```python
from build123d import *

# Parameters (mm, degrees)
SKETCH_1_R          = 18.5
SKETCH_1_R_2        = 6
EXTRUDE_1_DEPTH     = 14
SKETCH_2_R          = 18.5
SKETCH_2_R_2        = 17.3
CUT_EXTRUDE_1_DEPTH = 2.2
SKETCH_2_2_R        = 18.5
SKETCH_2_2_R_2      = 17.3
CUT_EXTRUDE_2_DEPTH = 0.8
SKETCH_2_4_R        = 18.5
SKETCH_2_4_R_2      = 17.3
CUT_EXTRUDE_3_DEPTH = 4
SKETCH_2_6_R        = 18.5
SKETCH_2_6_R_2      = 17.3
CUT_EXTRUDE_5_DEPTH = 3


with BuildPart() as part:
    # Sketch 1 → Extrude 1 (new body)
    with BuildSketch(Plane.XY):
        Circle(SKETCH_1_R)
        Circle(SKETCH_1_R_2, mode=Mode.SUBTRACT)
    extrude(amount=EXTRUDE_1_DEPTH)

    # Sketch 2 → Cut-Extrude 1 (cut)
    with BuildSketch(Plane.XY.offset(7.7)):
        Circle(SKETCH_2_R)
        Circle(SKETCH_2_R_2, mode=Mode.SUBTRACT)
    extrude(amount=-CUT_EXTRUDE_1_DEPTH, mode=Mode.SUBTRACT)

    # Sketch 2_2 → Cut-Extrude 2 (cut)
    with BuildSketch(Plane.XY.offset(7.7)):
        Circle(SKETCH_2_2_R)
        Circle(SKETCH_2_2_R_2, mode=Mode.SUBTRACT)
    extrude(amount=CUT_EXTRUDE_2_DEPTH, mode=Mode.SUBTRACT)

    # Sketch 2_4 → Cut-Extrude 3 (cut)
    with BuildSketch(Plane.XY.offset(7.7)):
        Circle(SKETCH_2_4_R)
        Circle(SKETCH_2_4_R_2, mode=Mode.SUBTRACT)
    extrude(amount=-CUT_EXTRUDE_3_DEPTH, mode=Mode.SUBTRACT)

    # Sketch 2_6 → Cut-Extrude 5 (cut)
    with BuildSketch(Plane.XY.offset(7.7)):
        Circle(SKETCH_2_6_R)
        Circle(SKETCH_2_6_R_2, mode=Mode.SUBTRACT)
    extrude(amount=CUT_EXTRUDE_5_DEPTH, mode=Mode.SUBTRACT)


solid = part.part
```
Part model, mm, in its own coordinate system. A direction names the side the tool comes from. Round coordinates to 2 decimals unless told otherwise and drop trailing zeros. Loops run counter-clockwise (first coordinate to the right, second up) from the corner with the lowest first, then second, coordinate; pieces in that order, holes last. Notation, with made-up numbers: (7, 65) -> (58, 65) arc R25 cw to (58, 85) -> close; hole circle Ø8 at (-32.5, 38.5). An arc over 180 degrees is marked (long way). Use CSV: the item, a comma, the result in double quotes. Start each with the question number.
1) Wall check: L1, parallel to Z at x = 8, y = 15.5; L2, parallel to Y at x = 0, z = 6.75; L3, parallel to Y at x = 0, z = 11. Give the ranges that are in metal, low to high. Write a range as [from, to].
2) Cut at D-D, the plane x = 9.5. Write the cut outline in (y, z).
3) Cut at C-C, the plane z = 9. Write the cut outline in (x, y), plus the area to 3 significant figures.
4) Which spindle directions (+Z, -Z, +X, -X, +Y, -Y) get a long thin tool onto all of the face, cutting with end or side? Do faces 1 (the flat face through (11, -14, 3.7)), 2 (the flat face through (-4.4, 4.4, 0)). Say none if no direction does.
5) Cut at A-A, the plane y = 0. Write the cut outline in (x, z), plus the area to 3 significant figures.
6) Drop flat-ended pins along their axis: P1, Ø3, axis at x = -13.5, z = 8, coming from the -Y side; P2, Ø1, axis at y = -14.5, z = 5.5, coming from the +X side; P3, Ø6, axis at y = -8.5, z = 4, coming from the -X side. Give the stop position or say it passes through.
7) Pull direction X, two halves, no side cores. Call faces 3 (the cylindrical face through (-4.01, -18.06, 12.33)), 4 (the cylindrical face through (-6, 0, 7)), 5 (the flat face through (11, -14, 10.7)): +X half, -X half, draft (parallel to the pull), parting line (faces both ways), or undercut.
Determined:
1,L1,"z = [0, 3.7], [10.7, 14]"
1,L2,"y = [-17.3, -6], [6, 17.3]"
1,L3,"y = [-18.5, -6], [6, 18.5]"
2,outline,"(-15.87, 0) -> (15.87, 0) -> (15.87, 3.7) -> (14.46, 3.7) -> (14.46, 10.7) -> (15.87, 10.7) -> (15.87, 14) -> (-15.87, 14) -> (-15.87, 10.7) -> (-14.46, 10.7) -> (-14.46, 3.7) -> (-15.87, 3.7) -> close"
3,outline,"circle Ø34.6 at (0, 0); hole circle Ø12 at (0, 0)"
3,area,"827 mm2"
4,face 1,"none"
4,face 2,"-Z, +X, -X, +Y, -Y"
5,outline,"(-18.5, 0) -> (-6, 0) -> (-6, 14) -> (-18.5, 14) -> (-18.5, 10.7) -> (-17.3, 10.7) -> (-17.3, 3.7) -> (-18.5, 3.7) -> close; (6, 0) -> (18.5, 0) -> (18.5, 3.7) -> (17.3, 3.7) -> (17.3, 10.7) -> (18.5, 10.7) -> (18.5, 14) -> (6, 14) -> close"
5,area,"333 mm2"
6,P1,"stops at y = -12.46"
6,P2,"stops at x = 10.16"
6,P3,"stops at x = -17.66"
7,face 3,"parting line"
7,face 4,"undercut"
7,face 5,"draft"
